Could you check a few things on this model? Use its own coordinates, in mm. A direction names the side the tool comes from. Give positions to 0.01 mm unless a question says otherwise; leave off trailing zeros. Loops run counter-clockwise (first coordinate to the right, second up) from the corner with the lowest first, then second, coordinate; pieces in that order, holes last. Notation, with made-up numbers: (62.25, 81) - (77.25, 81) arc R25 ccw to (77.25, 112) - close; hole circle Ø3 at (18.5, 87.25). An arc over 180 degrees is marked (long way). Use CSV: the item, a comma, the result in double quotes.
from build123d import *

# Parameters (mm, degrees)
F0_R          = 5.55625
F1_DEPTH      = 52
F1_DEPTH_BACK = 52
F2_R          = 4.7625
F3_DEPTH      = 61.5
F3_DEPTH_BACK = 61.5
F4_R          = 1.2
F5_DEPTH      = 5.55725
F5_DEPTH_BACK = 5.55725


with BuildPart() as f1:
    # F0 (on Right) → F1 (new body, two sides)
    with BuildSketch(Plane.YZ) as f1_sk:
        Circle(F0_R)
    extrude(amount=F1_DEPTH)
    extrude(f1_sk.sketch, amount=-F1_DEPTH_BACK)

    # F2 (on Right) → F3 (join, two sides)
    with BuildSketch(Plane.YZ) as f3_sk:
        Circle(F2_R)
    extrude(amount=F3_DEPTH)
    extrude(f3_sk.sketch, amount=-F3_DEPTH_BACK)

    # F4 (on Top) → F5 (cut, two sides)
    with BuildSketch(Plane.XY) as f5_sk:
        with Locations((-56.8, 0)):
            Circle(F4_R)
        with Locations((56.8, 0)):
            Circle(F4_R)
    extrude(amount=-F5_DEPTH, mode=Mode.SUBTRACT)
    extrude(f5_sk.sketch, amount=F5_DEPTH_BACK, mode=Mode.SUBTRACT)


solid = f1.part
1) I'm going to push flat-ended pins straight in: P1, Ø4, axis at x = 56.8, y = 0, coming from the +Z side; P2, Ø1, axis at x = 38, z = 2.5, coming from the +Y side; P3, Ø5, axis at x = 15, z = 4, coming from the -Y side. Where does each tip first touch, or does it pass through?
Answer below:
P1,"stops at z = 4.76"
P2,"stops at y = 5.18"
P3,"stops at y = -5.35"
2) Suppose I cut it at C-C (x = -56.8). Please give me the cut outline in (y, z) (1 decimal), plus the area to 3 significant figures.
Answer below:
outline,"(-1.2, -4.6) - (-1.2, 4.6) arc R4.8 ccw to start; (1.2, -4.6) arc R4.8 ccw to (1.2, 4.6) - close"
area,"48.6 mm2"
3) Suppose I cut it at A-A (y = 0). Please give me the cut outline in (x, z), plus the area to 3 significant figures.
Answer below:
outline,"(-61.5, -4.76) - (-58, -4.76) - (-58, 4.76) - (-61.5, 4.76) - close; (-55.6, -4.76) - (-52, -4.76) - (-52, -5.56) - (52, -5.56) - (52, -4.76) - (55.6, -4.76) - (55.6, 4.76) - (52, 4.76) - (52, 5.56) - (-52, 5.56) - (-52, 4.76) - (-55.6, 4.76) - close; (58, -4.76) - (61.5, -4.76) - (61.5, 4.76) - (58, 4.76) - close"
area,"1,290 mm2"
4) I need wall thicknesses on line 1 along X through (y, z) = (0, 3.25); line 2 along X through (y, z) = (-0.75, -3.75); line 3 along Y through (x, z) = (-56.8, 1.65). Which ranges of each line are inside material? Lowest first, please.
Answer below:
line 1,"x = -61.5 to -58, -55.6 to 55.6, 58 to 61.5"
line 2,"x = -61.5 to -57.74, -55.86 to 55.86, 57.74 to 61.5"
line 3,"y = -4.47 to -1.2, 1.2 to 4.47"
5) Which directions (+Z, -Z, +X, -X, +Y, -Y) give clear straight access to the entire face, cutting with the end or side of a thin tool? Please do faces 1 (the flat face through (-52, 5, 2)), 2 (the cylindrical face through (56.684, 2.198, -4.225)), 3 (the flat face through (61.5, 0, 0)).
Answer below:
face 1,"-X"
face 2,"+X"
face 3,"+Z, -Z, +X, +Y, -Y"
6) Suppose I cut it at D-D (x = 25.5). Please give me the cut outline in (y, z).
Answer below:
outline,"circle Ø11.11 at (0, 0)"
7) Suppose I cut it at B-B (z = 2.25). Please give me the cut outline in (x, y), plus the area to 3 significant figures.
Answer below:
outline,"(-61.5, -4.2) - (-52, -4.2) - (-52, -5.08) - (52, -5.08) - (52, -4.2) - (61.5, -4.2) - (61.5, 4.2) - (52, 4.2) - (52, 5.08) - (-52, 5.08) - (-52, 4.2) - (-61.5, 4.2) - close; hole circle Ø2.4 at (-56.8, 0); hole circle Ø2.4 at (56.8, 0)"
area,"1,210 mm2"
